Build history of the part. All positions in model axes, mm. A direction names the side the tool comes from. Coordinates: 2 decimals unless noted, no trailing zeros. Loops run counter-clockwise (first coordinate to the right, second up) from the corner with the lowest first, then second, coordinate; pieces in that order, holes last.
Item 1: Flat gauge pins, fed straight in: pin 1 (1.7 mm diameter, centred on y = 0.5, z = 9.5, fed in from +X); pin 2 (0.8 mm diameter, centred on x = 4, z = 16.5, fed in from -Y); pin 3 (1.2 mm diameter, centred on x = 0.5, z = 6.5, fed in from +Y). Where does each tip first touch, or does it go through?
Item 2: Cut at A-A (z = 11.25). List the corners of the cut face in (x, y), and give its area (3 significant figures).
Item 3: Cut at B-B (x = 3.75). List the corners of the cut face in (y, z).
Item 4: Cut at C-C (y = 4.6). List the corners of the cut face in (x, z), and give its area (3 significant figures).
Item 5: 3-axis set-ups, long thin cutter, end or side, ignore diameter. For faces 1 (the face through (4, 1.5, 12)), 2 (the face through (1, 1.5, 12)), 3 (the face through (4, 3.5, 12)): which of +Z, -Z, +X, -X, +Y, -Y reach the whole face in a straight line?
Item 6: Drill centre lines: line 1 along Y through (x, z) = (0.8, 21.5); line 2 along Z through (x, y) = (3.45, 0.9). Where is each one in solid material? Low to high.
from build123d import *

# Parameters (mm, degrees)
SKETCH1_W           = 5
SKETCH1_H           = 5
BOSS_EXTRUDE1_DEPTH = 24
SKETCH2_W           = 1.5
SKETCH2_H           = 1.5
CUT_EXTRUDE1_DEPTH  = 26.019992006
FILLET1_R           = 1
FILLET2_R           = 1


with BuildPart() as part:
    # Sketch1 → Boss-Extrude1 (new body)
    with BuildSketch(Plane.XY):
        with Locations((2.5, 2.5)):
            Rectangle(SKETCH1_W, SKETCH1_H)
    extrude(amount=BOSS_EXTRUDE1_DEPTH)

    # Sketch2 → Cut-Extrude1 (cut, through all)
    with BuildSketch(Plane.XY.offset(24)):
        with Locations((0.75, 4.25)):
            Rectangle(SKETCH2_W, SKETCH2_H)
        with Locations((4.25, 4.25)):
            Rectangle(SKETCH2_W, SKETCH2_H)
        with Locations((4.25, 0.75)):
            Rectangle(SKETCH2_W, SKETCH2_H)
        with Locations((0.75, 0.75)):
            Rectangle(SKETCH2_W, SKETCH2_H)
    extrude(amount=-CUT_EXTRUDE1_DEPTH, mode=Mode.SUBTRACT)

    # Fillet1
    fillet1_edges = [part.edges().sort_by_distance(p)[0] for p in [
        (0, 2.5, 24),
        (2.5, 5, 24),
        (5, 2.5, 24),
        (2.5, 0, 24),
    ]]
    fillet(fillet1_edges, radius=FILLET1_R)

    # Fillet2
    fillet2_edges = [part.edges().sort_by_distance(p)[0] for p in [
        (0, 2.5, 0),
        (2.5, 5, 0),
        (5, 2.5, 0),
        (2.5, 0, 0),
    ]]
    fillet(fillet2_edges, radius=FILLET2_R)


solid = part.part
Filled sheet:
1. pin 1: stops at x = 3.5
1. pin 2: stops at y = 1.5
1. pin 3: stops at y = 3.5
2. outline: (0, 1.5) - (1.5, 1.5) - (1.5, 0) - (3.5, 0) - (3.5, 1.5) - (5, 1.5) - (5, 3.5) - (3.5, 3.5) - (3.5, 5) - (1.5, 5) - (1.5, 3.5) - (0, 3.5) - close
2. area: 16.0 mm2
3. outline: (1.5, 0) - (3.5, 0) - (3.5, 24) - (1.5, 24) - close
4. outline: (1.5, 0.2) - (3.5, 0.2) - (3.5, 23.8) - (1.5, 23.8) - close
4. area: 47.2 mm2
5. face 1: +Z, -Z, +X, -Y
5. face 2: +Z, -Z, -X, -Y
5. face 3: +Z, -Z, +X, +Y
6. line 1: y = 1.5 to 3.5
6. line 2: z = 0.01 to 23.99
